Design review of the part built by this model. Coordinates are the model's own, in mm. Round coordinates to 2 decimals unless told otherwise and drop trailing zeros. Write each loop counter-clockwise with the first axis right and the second up, starting at its lowest first coordinate (ties: lowest second). Pieces come first, ordered by that corner, then holes. Notation, with made-up numbers: (63.25, -12) -> (99.25, -12) arc R24 ccw to (99.25, -2) -> close; hole circle Ø11 at (74.5, 40.25). An arc over 180 degrees is marked (long way). One line per question, with ' | ' between items. Start each with the question number.
1) Consider section A-A (x = 101). Give the boundary of the cut face in (y, z).
2) For probe 1 along X at (y, z) = (1.75, 9); probe 2 along X at (y, z) = (3.6, -104); probe 3 along Z at (x, y) = (37.5, 3), list the stretches that pass through material, from the lowest coordinate up.
3) Consider section B-B (z = -38.5). Give the boundary of the cut face in (x, y).
4) Insertion check: pin 1 Ø1.2 at (y, z) = (2, 58) entering from -X; pin 2 Ø2 at (x, y) = (70, 3.5) entering from -Z; pin 3 Ø2 at (x, y) = (120.5, 1.5) entering from +Z. Each pin has a flat end and moves straight along its axis. Give the tip position at first contact, or say it passes through.
Autodesk Inventor part; units mm, degrees
ref_plane "YZ Plane" through (0, 0, 0) normal (1, 0, 0) x (0, 1, 0)
ref_plane "XZ Plane" through (0, 0, 0) normal (0, 1, 0) x (-1, 0, 0)
ref_plane "XY Plane" through (0, 0, 0) normal (0, 0, 1) x (1, 0, 0)
sketch "Sketch1" plane through (0, 0, 0) normal (0, 1, 0) x (-1, 0, 0)
  line L0 (58.4588, 59.1887) -> (-121.5412, 59.1887)
  line L1 (-121.5412, -240.8113) -> (58.4588, -240.8113)
  line L2 (58.4588, -240.8113) -> (58.4588, 59.1887)
  line L3 (-121.5412, 59.1887) -> (-121.5412, -240.8113)
  line L4 (58.4588, 59.1887) -> (54.4588, 59.1887)
  line L5 (54.4588, 59.1887) -> (54.4588, 44.1887)
  line L6 (54.4588, 44.1887) -> (58.4588, 44.1887)
  line L7 (58.4588, 44.1887) -> (58.4588, 59.1887)
  line L8 (54.4588, 29.1887) -> (54.4588, 14.1887)
  line L9 (54.4588, 14.1887) -> (58.4588, 14.1887)
  line L10 (58.4588, 29.1887) -> (54.4588, 29.1887)
  line L11 (54.4588, -0.8113) -> (54.4588, -15.8113)
  line L12 (54.4588, -15.8113) -> (58.4588, -15.8113)
  line L13 (58.4588, -0.8113) -> (54.4588, -0.8113)
  line L14 (54.4588, -30.8113) -> (54.4588, -45.8113)
  line L15 (54.4588, -45.8113) -> (58.4588, -45.8113)
  line L16 (58.4588, -30.8113) -> (54.4588, -30.8113)
  line L17 (54.4588, -60.8113) -> (54.4588, -75.8113)
  line L18 (54.4588, -75.8113) -> (58.4588, -75.8113)
  line L19 (58.4588, -60.8113) -> (54.4588, -60.8113)
  line L20 (54.4588, -90.8113) -> (54.4588, -105.8113)
  line L21 (54.4588, -105.8113) -> (58.4588, -105.8113)
  line L22 (58.4588, -90.8113) -> (54.4588, -90.8113)
  line L23 (54.4588, -120.8113) -> (54.4588, -135.8113)
  line L24 (54.4588, -135.8113) -> (58.4588, -135.8113)
  line L25 (58.4588, -120.8113) -> (54.4588, -120.8113)
  line L26 (54.4588, -150.8113) -> (54.4588, -165.8113)
  line L27 (54.4588, -165.8113) -> (58.4588, -165.8113)
  line L28 (58.4588, -150.8113) -> (54.4588, -150.8113)
  line L29 (54.4588, -180.8113) -> (54.4588, -195.8113)
  line L30 (54.4588, -195.8113) -> (58.4588, -195.8113)
  line L31 (58.4588, -180.8113) -> (54.4588, -180.8113)
  line L32 (54.4588, -210.8113) -> (54.4588, -225.8113)
  line L33 (54.4588, -225.8113) -> (58.4588, -225.8113)
  line L34 (58.4588, -210.8113) -> (54.4588, -210.8113)
  line L35 (-121.5412, -240.8113) -> (-117.5412, -240.8113)
  line L36 (-117.5412, -240.8113) -> (-117.5412, -225.8113)
  line L37 (-117.5412, -225.8113) -> (-121.5412, -225.8113)
  line L38 (-121.5412, -225.8113) -> (-121.5412, -240.8113)
  line L39 (-117.5412, -210.8113) -> (-117.5412, -195.8113)
  line L40 (-117.5412, -195.8113) -> (-121.5412, -195.8113)
  line L41 (-121.5412, -210.8113) -> (-117.5412, -210.8113)
  line L42 (-117.5412, -180.8113) -> (-117.5412, -165.8113)
  line L43 (-117.5412, -165.8113) -> (-121.5412, -165.8113)
  line L44 (-121.5412, -180.8113) -> (-117.5412, -180.8113)
  line L45 (-117.5412, -150.8113) -> (-117.5412, -135.8113)
  line L46 (-117.5412, -135.8113) -> (-121.5412, -135.8113)
  line L47 (-121.5412, -150.8113) -> (-117.5412, -150.8113)
  line L48 (-117.5412, -120.8113) -> (-117.5412, -105.8113)
  line L49 (-117.5412, -105.8113) -> (-121.5412, -105.8113)
  line L50 (-121.5412, -120.8113) -> (-117.5412, -120.8113)
  line L51 (-117.5412, -90.8113) -> (-117.5412, -75.8113)
  line L52 (-117.5412, -75.8113) -> (-121.5412, -75.8113)
  line L53 (-121.5412, -90.8113) -> (-117.5412, -90.8113)
  line L54 (-117.5412, -60.8113) -> (-117.5412, -45.8113)
  line L55 (-117.5412, -45.8113) -> (-121.5412, -45.8113)
  line L56 (-121.5412, -60.8113) -> (-117.5412, -60.8113)
  line L57 (-117.5412, -30.8113) -> (-117.5412, -15.8113)
  line L58 (-117.5412, -15.8113) -> (-121.5412, -15.8113)
  line L59 (-121.5412, -30.8113) -> (-117.5412, -30.8113)
  line L60 (-117.5412, -0.8113) -> (-117.5412, 14.1887)
  line L61 (-117.5412, 14.1887) -> (-121.5412, 14.1887)
  line L62 (-121.5412, -0.8113) -> (-117.5412, -0.8113)
  line L63 (-117.5412, 29.1887) -> (-117.5412, 44.1887)
  line L64 (-117.5412, 44.1887) -> (-121.5412, 44.1887)
  line L65 (-121.5412, 29.1887) -> (-117.5412, 29.1887)
  line L66 (58.4588, -240.8113) -> (43.4588, -240.8113)
  line L67 (43.4588, -240.8113) -> (43.4588, -236.8113)
  line L68 (43.4588, -236.8113) -> (58.4588, -236.8113)
  line L69 (58.4588, -236.8113) -> (58.4588, -240.8113)
  line L70 (13.4588, -236.8113) -> (28.4588, -236.8113)
  line L71 (13.4588, -240.8113) -> (13.4588, -236.8113)
  line L72 (28.4588, -236.8113) -> (28.4588, -240.8113)
  line L73 (-16.5412, -236.8113) -> (-1.5412, -236.8113)
  line L74 (-16.5412, -240.8113) -> (-16.5412, -236.8113)
  line L75 (-1.5412, -236.8113) -> (-1.5412, -240.8113)
  line L76 (-46.5412, -236.8113) -> (-31.5412, -236.8113)
  line L77 (-46.5412, -240.8113) -> (-46.5412, -236.8113)
  line L78 (-31.5412, -236.8113) -> (-31.5412, -240.8113)
  line L79 (-76.5412, -236.8113) -> (-61.5412, -236.8113)
  line L80 (-76.5412, -240.8113) -> (-76.5412, -236.8113)
  line L81 (-61.5412, -236.8113) -> (-61.5412, -240.8113)
  line L82 (-106.5412, -236.8113) -> (-91.5412, -236.8113)
  line L83 (-106.5412, -240.8113) -> (-106.5412, -236.8113)
  line L84 (-91.5412, -236.8113) -> (-91.5412, -240.8113)
  line L85 (-121.5412, 59.1887) -> (-106.5412, 59.1887)
  line L86 (-106.5412, 59.1887) -> (-106.5412, 55.1887)
  line L87 (-106.5412, 55.1887) -> (-121.5412, 55.1887)
  line L88 (-121.5412, 55.1887) -> (-121.5412, 59.1887)
  line L89 (-76.5412, 59.1887) -> (-76.5412, 55.1887)
  line L90 (-76.5412, 55.1887) -> (-91.5412, 55.1887)
  line L91 (-91.5412, 55.1887) -> (-91.5412, 59.1887)
  line L92 (-46.5412, 59.1887) -> (-46.5412, 55.1887)
  line L93 (-46.5412, 55.1887) -> (-61.5412, 55.1887)
  line L94 (-61.5412, 55.1887) -> (-61.5412, 59.1887)
  line L95 (-16.5412, 59.1887) -> (-16.5412, 55.1887)
  line L96 (-16.5412, 55.1887) -> (-31.5412, 55.1887)
  line L97 (-31.5412, 55.1887) -> (-31.5412, 59.1887)
  line L98 (13.4588, 59.1887) -> (13.4588, 55.1887)
  line L99 (13.4588, 55.1887) -> (-1.5412, 55.1887)
  line L100 (-1.5412, 55.1887) -> (-1.5412, 59.1887)
  line L101 (43.4588, 59.1887) -> (43.4588, 55.1887)
  line L102 (43.4588, 55.1887) -> (28.4588, 55.1887)
  line L103 (28.4588, 55.1887) -> (28.4588, 59.1887)
  dimension "d22" = 4
  dimension "d23" = 15
  dimension "d26" = 30
  dimension "d31" = 4
  dimension "d32" = 15
  dimension "d35" = 30
  dimension "d40" = 15
  dimension "d41" = 4
  dimension "d44" = 30
  dimension "d49" = 15
  dimension "d50" = 4
  dimension "d53" = 30
extrude "Extrusion1" add sketch "Sketch1" along normal blind 4 contours L5 L6 L2 L10 L8 L9 L13 L11 L12 L16 L14 L15 L19 L17 L18 L22 L20 L21 L25 L23 L24 L28 L26 L27 L31 L29 L30 L34 L32 L33 L68 L67 L1 L72 L70 L71 L75 L73 L74 L78 L76 L77 L81 L79 L80 L84 L82 L83 L36 L37 L3 L41 L39 L40 L44 L42 L43 L47 L45 L46 L50 L48 L49 L53 L51 L52 L56 L54 L55 L59 L57 L58 L62 L60 L61 L65 L63 L64 L87 L86 L0 L91 L90 L89 L94 L93 L92 L97 L96 L95 L100 L99 L98 L103 L102 L101
sketch "Sketch2" plane through (0, 0, 0) normal (0, -1, 0) x (1, 0, 0)
  line L0 (-54.4588, 29.1887) -> (-58.4588, 29.1887)
  line L1 (-58.4588, 29.1887) -> (-58.4588, 44.1887)
  line L2 (-54.4588, 29.1887) -> (-58.4588, 29.1887)
  line L3 (-58.4588, 29.1887) -> (-58.4588, 44.1887)
  line L4 (-58.4588, 44.1887) -> (-54.4588, 44.1887)
  line L5 (-54.4588, 44.1887) -> (-54.4588, 29.1887)
  line L6 (91.5412, 59.1887) -> (106.5412, 59.1887)
  line L7 (91.5412, 59.1887) -> (106.5412, 59.1887)
  line L8 (106.5412, 59.1887) -> (106.5412, 55.1887)
  line L9 (106.5412, 55.1887) -> (91.5412, 55.1887)
  line L10 (91.5412, 55.1887) -> (91.5412, 59.1887)
  line L11 (117.5412, -225.8113) -> (117.5412, -240.8113)
  line L12 (106.5412, -236.8113) -> (91.5412, -236.8113)
  line L13 (117.5412, -240.8113) -> (106.5412, -240.8113)
  line L14 (106.5412, -240.8113) -> (106.5412, -236.8113)
  line L15 (106.5412, -236.8113) -> (117.5412, -236.8113)
  line L16 (117.5412, -236.8113) -> (117.5412, -240.8113)
  line L17 (121.5412, -225.8113) -> (117.5412, -225.8113)
  line L18 (121.5412, -210.8113) -> (121.5412, -225.8113)
  line L19 (117.5412, -225.8113) -> (121.5412, -225.8113)
  line L20 (121.5412, -225.8113) -> (121.5412, -210.8113)
  line L21 (121.5412, -210.8113) -> (117.5412, -210.8113)
  line L22 (117.5412, -210.8113) -> (117.5412, -225.8113)
  line L23 (-54.4588, -225.8113) -> (-54.4588, -210.8113)
  line L24 (-54.4588, -225.8113) -> (-58.4588, -225.8113)
  line L25 (-58.4588, -225.8113) -> (-58.4588, -236.8113)
  line L26 (-58.4588, -236.8113) -> (-54.4588, -236.8113)
  line L27 (-54.4588, -236.8113) -> (-54.4588, -225.8113)
  line L28 (-28.4588, -240.8113) -> (-43.4588, -240.8113)
  line L29 (-43.4588, -240.8113) -> (-43.4588, -236.8113)
  line L30 (-28.4588, -240.8113) -> (-43.4588, -240.8113)
  line L31 (-43.4588, -240.8113) -> (-43.4588, -236.8113)
  line L32 (-43.4588, -236.8113) -> (-28.4588, -236.8113)
  line L33 (-28.4588, -236.8113) -> (-28.4588, -240.8113)
  line L34 (121.5412, 55.1887) -> (121.5412, 44.1887)
  line L35 (121.5412, 44.1887) -> (117.5412, 44.1887)
  line L36 (121.5412, 55.1887) -> (117.5412, 55.1887)
  line L37 (117.5412, 55.1887) -> (117.5412, 44.1887)
  line L38 (117.5412, 44.1887) -> (121.5412, 44.1887)
  line L39 (121.5412, 44.1887) -> (121.5412, 55.1887)
  line L40 (-54.4588, 59.1887) -> (-43.4588, 59.1887)
  line L41 (-43.4588, 55.1887) -> (-28.4588, 55.1887)
  line L42 (-54.4588, 59.1887) -> (-43.4588, 59.1887)
  line L43 (-43.4588, 59.1887) -> (-43.4588, 55.1887)
  line L44 (-43.4588, 55.1887) -> (-54.4588, 55.1887)
  line L45 (-54.4588, 55.1887) -> (-54.4588, 59.1887)
  point P0 (0, 0)
extrude "Extrusion2" cut sketch "Sketch2" against normal through all
equation "\"d22\" = WoodThickness"
equation "\"d26\" = 2 * d23"
equation "\"d31\" = WoodThickness"
equation "\"d35\" = 2 * d32"
equation "\"d41\" = WoodThickness"
equation "\"d44\" = 2 * d40"
equation "\"d50\" = WoodThickness"
equation "\"d53\" = 2 * d49"
equation "\"d2\" = WoodThickness"
properties part number "ground"
From the geometry:
1) outline: (0, -236.81) -> (4, -236.81) -> (4, 55.19) -> (0, 55.19) -> close
2) probe 1: x = -58.46 to 117.54 | probe 2: x = -54.46 to 121.54 | probe 3: z = -236.81 to 59.19
3) outline: (-54.46, 0) -> (121.54, 0) -> (121.54, 4) -> (-54.46, 4) -> close
4) pin 1: stops at x = -28.46 | pin 2: stops at z = -236.81 | pin 3: stops at z = 29.19
